Could you check a few things on this model? Use its own coordinates, in mm. A direction names the side the tool comes from. Give positions to 0.01 mm unless a question says otherwise; leave off trailing zeros. Order: outer loops, then holes, each group sorted by start corner. A loop starts at its lowest first (then second) coordinate and runs counter-clockwise, first axis right, second up.
Autodesk Inventor part; units mm, degrees
ref_plane "YZ Plane" through (0, 0, 0) normal (1, 0, 0) x (0, 1, 0)
ref_plane "XZ Plane" through (0, 0, 0) normal (0, 1, 0) x (-1, 0, 0)
ref_plane "XY Plane" through (0, 0, 0) normal (0, 0, 1) x (1, 0, 0)
sketch "Boceto1" plane through (0, 0, 0) normal (0, 1, 0) x (-1, 0, 0)
  line L0 (5.1, 27.5) -> (-5.1, 27.5)
  line L1 (-5.1, 27.5) -> (-5.1, -27.5)
  line L2 (-5.1, -27.5) -> (5.1, -27.5)
  line L3 (5.1, -27.5) -> (5.1, 27.5)
  circle A0 centre (0, 0) radius 5.1
  line L4 (0, 0) -> (7.6193, 0) construction
  point P0 (-5.1, 0)
  dimension "d0" = 10.2
  dimension "d12" = 55
extrude "Extrusión1" add sketch "Boceto1" along normal blind 20 contours L3 A0 L1 L0 | L3 L2 L1 A0
sketch "Boceto2" plane through (0, 20, 0) normal (0, 1, 0) x (1, 0, 0)
  line L0 (-13.1, -27.5) -> (13.1, -27.5)
  line L1 (13.1, -27.5) -> (13.1, 27.5)
  line L2 (13.1, 27.5) -> (-13.1, 27.5)
  line L3 (-13.1, 27.5) -> (-13.1, -27.5)
  line L4 (-5.1, -27.5) -> (5.1, -27.5)
  line L5 (5.1, 27.5) -> (-5.1, 27.5)
  arc A0 (-5.1, 0) -> (5.1, 0) centre (0, 0) ccw
  line L6 (-5.1, 0) -> (-13.1, 0) construction
  circle A1 centre (0, 0) radius 5.1
  point P0 (0, -27.5)
  point P1 (0, 27.5)
  dimension "d3" = 8
extrude "Extrusión2" add sketch "Boceto2" along normal blind 10
sketch "Boceto3" plane through (0, 0, 0) normal (0, -1, 0) x (1, 0, 0)
  line L0 (-13.1982, 2) -> (11.7656, 2)
  line L1 (11.7656, 2) -> (11.7656, -2)
  line L2 (11.7656, -2) -> (-13.1982, -2)
  line L3 (-13.1982, -2) -> (-13.1982, 2)
  line L4 (0, 0) -> (-16.4322, 0) construction
  dimension "d6" = 4
extrude "Extrusión3" cut sketch "Boceto3" against normal up to surface (20 mm away)
chamfer "Chaflán1" distance 5 angle 45 2 edges at (13.1, 30, 0) (-13.1, 30, 0)
sketch "Boceto4" plane through (0, 20, 0) normal (0, -1, 0) x (1, 0, 0)
  line L0 (5.1, -27.5) -> (9.1, -27.5)
  line L1 (9.1, -27.5) -> (9.1, 27.5)
  line L2 (5.1, 27.5) -> (13.1, 27.5)
  line L3 (9.1, 27.5) -> (5.1, 27.5)
  line L4 (13.1, -27.5) -> (5.1, -27.5)
  line L5 (5.1, 27.5) -> (5.1, -27.5)
  line L6 (-5.1, -27.5) -> (-13.1, -27.5)
  line L7 (-5.1, -27.5) -> (-9.1, -27.5)
  line L8 (-5.1, 2) -> (-5.1, 27.5)
  line L9 (-5.1, 27.5) -> (-9.1, 27.5)
  line L10 (-13.1, 27.5) -> (-5.1, 27.5)
  line L11 (-9.1, 27.5) -> (-9.1, -27.5)
  line L12 (-5.1, -27.5) -> (-5.1, -2)
  line L13 (-5.1, 27.5) -> (-5.1, -27.5)
  point P0 (0, 0)
  dimension "d13" = 4
  dimension "d14" = 4
extrude "Extrusión4" cut sketch "Boceto4" against normal blind 4
properties part number "SoporteVarilla"
Item 1: Imagine slicing it at C-C on z = -18.5. List the corners of the cut face in (x, y) for me, then the cut area to 3 significant figures.
Findings:
outline: (-13.1, 20) - (-9.1, 20) - (-9.1, 24) - (-5.1, 24) - (-5.1, 0) - (5.1, 0) - (5.1, 24) - (9.1, 24) - (9.1, 20) - (13.1, 20) - (13.1, 25) - (8.1, 30) - (-8.1, 30) - (-13.1, 25) - close
area: 409 mm2
Item 2: Imagine slicing it at D-D on x = 7. List the corners of the cut face in (y, z) for me, then the cut area to 3 significant figures.
Findings:
outline: (24, -27.5) - (30, -27.5) - (30, 27.5) - (24, 27.5) - close
area: 330 mm2
Item 3: We'd pull the mould along X, two halves only. Please class faces 4 (the flat face through (-5.1, 12, 14)), 5 (the flat face through (13.1, 22, 0)), 6 (the flat face through (11, 20, 0)): +X half, -X half, draft (parallel to the pull), parting line (faces both ways), or undercut.
Findings:
face 4: undercut
face 5: +X half
face 6: draft
Item 4: For faces 1 (the flat face through (0, 18, -27.5)), 2 (the flat face through (-7, 24, 0)), 3 (the flat face through (-11, 20, 0)), which set-ups out of +Z, -Z, +X, -X, +Y, -Y let a thin tool reach every point of the face, with its end or its side?
Findings:
face 1: -Z, +X, -X, +Y, -Y
face 2: +Z, -Z, -Y
face 3: +Z, -Z, -X, -Y
Item 5: For pin 1 (1.5 mm diameter, centred on y = 9, z = -7, fed in from +X); pin 2 (12 mm diameter, centred on y = 7, z = -5.5, fed in from -X); pin 3 (1 mm diameter, centred on x = 7, y = 17, fed in from -Z); pin 4 (1.2 mm diameter, centred on x = 11.5, z = 6, fed in from -Y), each with a flat end and sliding along its axis, tell me the tip position at first contact or that it passes through.
Findings:
pin 1: stops at x = 5.1
pin 2: stops at x = -5.1
pin 3: passes through
pin 4: stops at y = 20
Item 6: Please list where these lines run through material, in increasing order: line 1 along X through (y, z) = (22.25, -18); line 2 along Z through (x, y) = (0, 19.25); line 3 along Y through (x, z) = (-7.5, 14.5).
Findings:
line 1: x = -13.1 to -9.1, -5.1 to 5.1, 9.1 to 13.1
line 2: z = -27.5 to -5.1, 5.1 to 27.5
line 3: y = 24 to 30
Item 7: Imagine slicing it at A-A on y = 17.5. List the corners of the cut face in (x, z) for me, then the cut area to 3 significant figures.
Findings:
outline: (-5.1, -27.5) - (5.1, -27.5) - (5.1, -2) - (4.69, -2) arc R5.1 cw to (-4.69, -2) - (-5.1, -2) - close; (-5.1, 2) - (-4.69, 2) arc R5.1 cw to (4.69, 2) - (5.1, 2) - (5.1, 27.5) - (-5.1, 27.5) - close
area: 478 mm2
Item 8: Imagine slicing it at B-B on x = 0. List the corners of the cut face in (y, z) for me, then the cut area to 3 significant figures.
Findings:
outline: (0, -27.5) - (30, -27.5) - (30, -5.1) - (0, -5.1) - close; (0, 5.1) - (30, 5.1) - (30, 27.5) - (0, 27.5) - close
area: 1,340 mm2
